Can you work these out from the model? Positions are in its coordinate system, mm. A direction names the side the tool comes from. Coordinates: 2 decimals unless noted, no trailing zeros. Loops run counter-clockwise (first coordinate to the right, second up) from the corner with the lowest first, then second, coordinate; pieces in that order, holes last. Notation, with made-up numbers: M 34,83.25 L 92,83.25 A17 cw 92,96.25 Z; hole C -38.5,-9 d10. An arc over 180 degrees is marked long. Answer as a JSON object with one key per item and string values. Group by question number.
Item 1: If I drill on line 1 (Y direction, x = 5.5, z = 12.5); line 2 (Y direction, x = 3.5, z = 12.5); line 3 (X direction, y = 23, z = 4), over which ranges is the centre line in solid material (lowest first)?
Item 2: Which directions (+Z, -Z, +X, -X, +Y, -Y) give clear straight access to the entire face, cutting with the end or side of a thin tool? Please do faces 4 (the flat face through (-7.74, 24, 12)), 5 (the flat face through (7.74, 24, 12)), 6 (the flat face through (-0.259, 20, 15)).
Item 3: Suppose I cut it at A-A (y = 0). Write out the boundary of the cut face in (x, z).
Item 4: I'm going to push flat-ended pins straight in: pin 1 Ø5 at (x, z) = (8.5, 3) entering from +Y; pin 2 Ø7 at (y, z) = (17, 10) entering from -X; pin 3 Ø1 at (x, z) = (1.5, 8.5) entering from +Y. Where does each tip first touch, or does it pass through?
Item 5: Suppose I cut it at B-B (x = -2.5). Write out the boundary of the cut face in (y, z).
Item 6: Suppose I cut it at D-D (x = 11.5). Write out the boundary of the cut face in (y, z).
Item 7: Suppose I cut it at C-C (z = 8). Write out the boundary of the cut face in (x, y).
Item 8: We'd pull the mould along Y, two halves only. Please class faces 1 (the cylindrical face through (4.08, 26.95, 12.32)), 2 (the cylindrical face through (-3.947, 19.565, 14.484)), 3 (the cylindrical face through (0, -16, 14)): +Y half, -Y half, draft (parallel to the pull), parting line (faces both ways), or undercut.
```python
from build123d import *

# Parameters (mm, degrees)
SKETCH_1_R          = 3.5
SKETCH_1_R_2        = 13
EXTRUDE_2_DEPTH     = 10
SKETCH_2_R          = 13
EXTRUDE_3_DEPTH     = 15
SKETCH_3_W          = 0.517195108
SKETCH_3_H          = 18.726193104
CUT_EXTRUDE_1_DEPTH = 26
SKETCH_4_R          = 2.5
CUT_EXTRUDE_2_DEPTH = 43.740275714
CUT_EXTRUDE_3_DEPTH = 11
SKETCH_6_R          = 1.5
CUT_EXTRUDE_4_DEPTH = 21


with BuildPart() as part:
    # 草图1 → 凸台-拉伸2 (new body)
    with BuildSketch(Plane.XY):
        with BuildLine():
            Line((-35, -7), (-7.740275714, -18.44147857))
            ThreePointArc((-7.740275714, -18.44147857), (0, -20), (7.740275714, -18.44147857))
            Line((7.740275714, -18.44147857), (35, -7))
            Line((35, -7), (35, 7))
            Line((35, 7), (7.740275714, 18.44147857))
            Line((7.740275714, 18.44147857), (7.740275714, 25.44147857))
            ThreePointArc((7.740275714, 25.44147857), (0, 27.494244152), (-7.740275714, 25.44147857))
            Line((-7.740275714, 25.44147857), (-7.740275714, 18.44147857))
            Line((-7.740275714, 18.44147857), (-35, 7))
            Line((-35, 7), (-35, -7))
        make_face()
        with Locations((-28, 0)):
            Circle(SKETCH_1_R, mode=Mode.SUBTRACT)
        Circle(SKETCH_1_R_2, mode=Mode.SUBTRACT)
        with Locations((28, 0)):
            Circle(SKETCH_1_R, mode=Mode.SUBTRACT)
    extrude(amount=EXTRUDE_2_DEPTH)

    # 草图2 → 凸台-拉伸3 (add)
    with BuildSketch(Plane.XY.offset(10)):
        with BuildLine():
            Line((-7.740275714, 18.44147857), (-7.740275714, 25.44147857))
            ThreePointArc((-7.740275714, 25.44147857), (0, 27.494244152), (7.740275714, 25.44147857))
            Line((7.740275714, 25.44147857), (7.740275714, 18.44147857))
            ThreePointArc((7.740275714, 18.44147857), (0, -20), (-7.740275714, 18.44147857))
        make_face()
        Circle(SKETCH_2_R, mode=Mode.SUBTRACT)
    extrude(amount=EXTRUDE_3_DEPTH)

    # 草图3 → 切除-拉伸1 (cut, through all)
    with BuildSketch(Plane.XY.offset(25)):
        with Locations((0, 21.741202931)):
            Rectangle(SKETCH_3_W, SKETCH_3_H)
    extrude(amount=-CUT_EXTRUDE_1_DEPTH, mode=Mode.SUBTRACT)

    # 草图4 → 切除-拉伸2 (cut, through all)
    with BuildSketch(Plane(origin=(7.740275714, 0, 0), x_dir=(0, 0, -1), z_dir=(1, 0, 0))):
        with Locations((-12.5, 21.086423576)):
            Circle(SKETCH_4_R)
    extrude(amount=-CUT_EXTRUDE_2_DEPTH, mode=Mode.SUBTRACT)

    # 草图5 → 切除-拉伸3 (cut, through all)
    with BuildSketch(Plane.XY.offset(10)):
        with BuildLine():
            Line((-7.740275714, 18.44147857), (-35, 7))
            Line((-35, 7), (-35, -7))
            Line((-35, -7), (-7.740275714, -18.44147857))
            ThreePointArc((-7.740275714, -18.44147857), (-20, 0), (-7.740275714, 18.44147857))
        make_face()
        with BuildLine():
            Line((7.740275714, 18.44147857), (35, 7))
            Line((35, 7), (35, -7))
            Line((35, -7), (7.740275714, -18.44147857))
            ThreePointArc((7.740275714, -18.44147857), (20, 0), (7.740275714, 18.44147857))
        make_face()
    extrude(amount=-CUT_EXTRUDE_3_DEPTH, mode=Mode.SUBTRACT)

    # 草图6 → 切除-拉伸4 (cut, through all)
    with BuildSketch(Plane(origin=(0, 0, 0), x_dir=(1, 0, 0), z_dir=(0, 1, 0))):
        with Locations((0, -12.5)):
            Circle(SKETCH_6_R)
    extrude(amount=-CUT_EXTRUDE_4_DEPTH, mode=Mode.SUBTRACT)


solid = part.part
```
From the geometry:
{
 "1": {"line 1": "-19.23 to -11.78, 11.78 to 18.59, 23.59 to 26.49", "line 2": "-19.69 to -12.52, 12.52 to 18.59, 23.59 to 27.1", "line 3": "-7.74 to -0.26, 0.26 to 7.74"},
 "2": {"face 4": "+Z, -Z, -X, +Y", "face 5": "+Z, -Z, +X, +Y", "face 6": "+Z, -Z, +Y"},
 "3": {"outline": "M -20,0 L -13,0 L -13,25 L -20,25 Z; M 13,0 L 20,0 L 20,25 L 13,25 Z"},
 "4": {"pin 1": "y = 26.3", "pin 2": "x = -14.76", "pin 3": "y = 27.46"},
 "5": {"outline": "M -19.84,0 L -12.76,0 L -12.76,25 L -19.84,25 Z; M 12.76,0 L 27.29,0 L 27.29,25 L 12.76,25 Z; hole C 21.09,12.5 d5"},
 "6": {"outline": "M -16.36,0 L -6.06,0 L -6.06,25 L -16.36,25 Z; M 6.06,0 L 16.36,0 L 16.36,25 L 6.06,25 Z"},
 "7": {"outline": "M -7.74,18.44 A20 ccw long 7.74,18.44 L 7.74,25.44 A15.62 ccw 0.26,27.49 L 0.26,13 A13 cw long -0.26,13 L -0.26,27.49 A15.62 ccw -7.74,25.44 Z"},
 "8": {"face 1": "+Y half", "face 2": "undercut", "face 3": "draft"}
}
